The model under review builds one solid part; all positions refer to its coordinate system, in mm. A direction names the side the tool comes from. Coordinates: 2 decimals unless noted, no trailing zeros. Loops run counter-clockwise (first coordinate to the right, second up) from the corner with the lowest first, then second, coordinate; pieces in that order, holes last. Notation, with made-up numbers: (-14, 4) - (26, 4) arc R33 cw to (26, 33) - close; hole circle Ø10 at (67, 86.5). An arc over 180 degrees is marked (long way). Use a Markdown table: item, result. Add a question column.
1) Add section B-B, the plane z = -11.5. Give the boundary of the cut face in (x, y), and give its area (3 significant figures).
2) Clearance check with flat-ended pins moving along their axes: pin 1 (3 mm diameter, centred on y = 13, z = -13, fed in from +X); pin 2 (0.5 mm diameter, centred on y = 27, z = 1, fed in from -X); pin 3 (0.9 mm diameter, centred on y = 28, z = 1, fed in from +X). State where each tip first meets the part, or that it passes through.
3) To check wall thickness, follow L1, parallel to Y at x = 20.5, z = 13; L2, parallel to Z at x = 22, y = 11; L3, parallel to X at y = 32, z = -12.5. State the ranges of each line that lie inside material, in increasing order. Write a range as [from, to].
4) The part is to be moulded in two halves that separate along X. For faces 1 (the flat face through (26.5, 20, 13)), 2 (the cylindrical face through (-11.54, 19.72, 9.89)), 3 (the flat face through (-21, 20, 11.1)), say which applies: pulls with the +X half, pulls with the -X half, needs draft (parallel to the pull), parting line crosses it, or undercut.
5) For faces 4 (the cylindrical face through (-0.332, 19.72, -15.096)), 5 (the flat face through (-16.5, 20, 5)), 6 (the flat face through (21, 20, 11.1)), 7 (the flat face through (6, 40, 14.4)), 8 (the flat face through (-26.5, 20, 13)), list the 3-axis set-ups (+Z, -Z, +X, -X, +Y, -Y) from which the entire face can be reached by the end or side of a thin tool; tool diameter is ignored.
6) Add section D-D, the plane y = 30.5. Give the boundary of the cut face in (x, z).
7) Add section C-C, the plane y = 6. Give the boundary of the cut face in (x, z), and give its area (3 significant figures).
8) Add section A-A, the plane x = -14.5. Give the boundary of the cut face in (y, z).
```python
from build123d import *

# Parameters (mm, degrees)
BOSS_EXTRUDE3_DEPTH = 40
SKETCH8_W           = 4
SKETCH8_H           = 40
BOSS_EXTRUDE6_DEPTH = 10
SKETCH9_W           = 4
SKETCH9_H           = 40
BOSS_EXTRUDE7_DEPTH = 10
BOSS_EXTRUDE9_DEPTH = 40
CUT_EXTRUDE1_DEPTH  = 40


with BuildPart() as part:
    # Sketch3 → Boss-Extrude3 (new body)
    with BuildSketch(Plane(origin=(0, 0, 0), x_dir=(1, 0, 0), z_dir=(0, 1, 0))):
        with BuildLine():
            ThreePointArc((16.5, 0), (0, 16.5), (-16.5, 0))
            Line((-16.5, 0), (-16.5, -15.1))
            Line((-16.5, -15.1), (-15.1, -15.1))
            Line((-15.1, -15.1), (-15.1, 0))
            ThreePointArc((-15.1, 0), (0, 15.1), (15.1, 0))
            Line((15.1, 0), (15.1, -15.1))
            Line((15.1, -15.1), (16.5, -15.1))
            Line((16.5, -15.1), (16.5, 0))
        make_face()
    extrude(amount=BOSS_EXTRUDE3_DEPTH)

    # Sketch8 → Boss-Extrude6 (add)
    with BuildSketch(Plane(origin=(16.5, 0, 0), x_dir=(0, 0, -1), z_dir=(1, 0, 0))):
        with Locations((-13.1, 20)):
            Rectangle(SKETCH8_W, SKETCH8_H)
    extrude(amount=BOSS_EXTRUDE6_DEPTH)

    # Sketch9 → Boss-Extrude7 (add)
    with BuildSketch(Plane.ZY.offset(16.5)):
        with Locations((13.1, 20)):
            Rectangle(SKETCH9_W, SKETCH9_H)
    extrude(amount=BOSS_EXTRUDE7_DEPTH)

    # Sketch10 → Boss-Extrude9 (add)
    with BuildSketch(Plane(origin=(0, 0, 0), x_dir=(-1, 0, 0), z_dir=(0, -1, 0))):
        with BuildLine():
            Line((3.791332709, -15.1), (15.1, -15.1))
            Line((15.1, -15.1), (15.1, -1.740689519))
            ThreePointArc((15.1, -1.740689519), (11.460081139, -9.985316234), (3.791332709, -14.719571879))
            Line((3.791332709, -14.719571879), (3.791332709, -15.1))
        make_face()
        with BuildLine():
            Line((-15.1, -15.1), (-3.791332709, -15.1))
            Line((-3.791332709, -15.1), (-3.791332709, -14.719571879))
            ThreePointArc((-3.791332709, -14.719571879), (-11.460081139, -9.985316234), (-15.1, -1.740689519))
            Line((-15.1, -1.740689519), (-15.1, -15.1))
        make_face()
    extrude(amount=-BOSS_EXTRUDE9_DEPTH)

    # Sketch11 → Cut-Extrude1 (cut)
    with BuildSketch(Plane(origin=(0, 0, 11.1), x_dir=(-1, 0, 0), z_dir=(0, 0, -1))):
        with BuildLine():
            ThreePointArc((-19.9, 33), (-20.36862915, 34.13137085), (-21.5, 34.6))
            Line((-21.5, 34.6), (-21.5, 31.4))
            ThreePointArc((-21.5, 31.4), (-20.36862915, 31.86862915), (-19.9, 33))
        make_face()
        with BuildLine():
            Line((-21.5, 31.4), (-21.5, 34.6))
            ThreePointArc((-21.5, 34.6), (-23.1, 33), (-21.5, 31.4))
        make_face()
        with BuildLine():
            ThreePointArc((-19.9, 7), (-20.36862915, 8.13137085), (-21.5, 8.6))
            Line((-21.5, 8.6), (-21.5, 5.4))
            ThreePointArc((-21.5, 5.4), (-20.36862915, 5.86862915), (-19.9, 7))
        make_face()
        with BuildLine():
            Line((-21.5, 5.4), (-21.5, 8.6))
            ThreePointArc((-21.5, 8.6), (-23.1, 7), (-21.5, 5.4))
        make_face()
        with BuildLine():
            ThreePointArc((23.1, 7), (22.63137085, 8.13137085), (21.5, 8.6))
            Line((21.5, 8.6), (21.5, 5.4))
            ThreePointArc((21.5, 5.4), (22.63137085, 5.86862915), (23.1, 7))
        make_face()
        with BuildLine():
            Line((21.5, 5.4), (21.5, 8.6))
            ThreePointArc((21.5, 8.6), (19.9, 7), (21.5, 5.4))
        make_face()
        with BuildLine():
            ThreePointArc((23.1, 33), (22.63137085, 34.13137085), (21.5, 34.6))
            Line((21.5, 34.6), (21.5, 31.4))
            ThreePointArc((21.5, 31.4), (22.63137085, 31.86862915), (23.1, 33))
        make_face()
        with BuildLine():
            Line((21.5, 31.4), (21.5, 34.6))
            ThreePointArc((21.5, 34.6), (19.9, 33), (21.5, 31.4))
        make_face()
    extrude(amount=-CUT_EXTRUDE1_DEPTH, mode=Mode.SUBTRACT)


solid = part.part
```
From the geometry:
| question | item | result |
|---|---|---|
| 1 | outline | (-11.83, 0) - (-9.79, 0) - (-9.79, 40) - (-11.83, 40) - close; (9.79, 0) - (11.83, 0) - (11.83, 40) - (9.79, 40) - close |
| 1 | area | 164 mm^2 |
| 2 | pin 1 | stops at x = 11.83 |
| 2 | pin 2 | stops at x = -16.5 |
| 2 | pin 3 | stops at x = 16.5 |
| 3 | L1 | y = [0, 5.75], [8.25, 31.75], [34.25, 40] |
| 3 | L2 | z = [11.1, 15.1] |
| 3 | L3 | x = [-10.77, -8.47], [8.47, 10.77] |
| 4 | face 1 | pulls with the +X half |
| 4 | face 2 | undercut |
| 4 | face 3 | needs draft |
| 5 | face 4 | +Y, -Y |
| 5 | face 5 | -Z, -X, +Y, -Y |
| 5 | face 6 | -Z, +X, +Y, -Y |
| 5 | face 7 | +Z, -Z, +X, -X, +Y |
| 5 | face 8 | +Z, -Z, -X, +Y, -Y |
| 6 | outline | (-26.5, 11.1) - (-16.5, 11.1) - (-16.5, 0) arc R16.5 ccw to (16.5, 0) - (16.5, 11.1) - (26.5, 11.1) - (26.5, 15.1) - (3.79, 15.1) - (3.79, 14.72) arc R15.2 cw to (15.1, 1.74) - (15.1, 0) arc R15.1 cw to (-15.1, 0) - (-15.1, 1.74) arc R15.2 cw to (-3.79, 14.72) - (-3.79, 15.1) - (-26.5, 15.1) - close |
| 7 | outline | (-26.5, 11.1) - (-22.75, 11.1) - (-22.75, 15.1) - (-26.5, 15.1) - close; (-20.25, 11.1) - (-16.5, 11.1) - (-16.5, 0) arc R16.5 ccw to (16.5, 0) - (16.5, 11.1) - (20.25, 11.1) - (20.25, 15.1) - (3.79, 15.1) - (3.79, 14.72) arc R15.2 cw to (15.1, 1.74) - (15.1, 0) arc R15.1 cw to (-15.1, 0) - (-15.1, 1.74) arc R15.2 cw to (-3.79, 14.72) - (-3.79, 15.1) - (-20.25, 15.1) - close; (22.75, 11.1) - (26.5, 11.1) - (26.5, 15.1) - (22.75, 15.1) - close |
| 7 | area | 265 mm^2 |
| 8 | outline | (0, -7.87) - (40, -7.87) - (40, -4.21) - (0, -4.21) - close; (0, 4.56) - (40, 4.56) - (40, 15.1) - (0, 15.1) - close |
